Build history of the part. All positions in model axes, mm. A direction names the side the tool comes from. Coordinates: 2 decimals unless noted, no trailing zeros. Order: outer loops, then holes, each group sorted by start corner. A loop starts at its lowest first (then second) coordinate and runs counter-clockwise, first axis right, second up. Notation, with made-up numbers: (71.5, 70.25) -> (110.5, 70.25) arc R23 cw to (110.5, 105.25) -> close; hole circle Ø11 at (-5.5, 25). An arc over 180 degrees is marked (long way). Write each question's results on one line, items separated by ' | '.
from build123d import *

# Parameters (mm, degrees)
EXTRUDE_1_DEPTH = 21.5
SKETCH_2_W      = 9.5
SKETCH_2_H      = 12
EXTRUDE_2_DEPTH = 5
SKETCH_3_W      = 10
SKETCH_3_H      = 12
EXTRUDE_3_DEPTH = 9
SKETCH_4_R      = 2
EXTRUDE_4_DEPTH = 0.7
EXTRUDE_6_DEPTH = 9.3


with BuildPart() as part:
    # 草图1 → 凸台-拉伸1 (new body)
    with BuildSketch(Plane(origin=(0, 0, 0), x_dir=(1, 0, 0), z_dir=(0, 1, 0))):
        with BuildLine():
            Line((-5, -3.31662479), (-5, 3.31662479))
            ThreePointArc((-5, 3.31662479), (0, 6), (5, 3.31662479))
            Line((5, 3.31662479), (5, -3.31662479))
            ThreePointArc((5, -3.31662479), (0, -6), (-5, -3.31662479))
        make_face()
    extrude(amount=EXTRUDE_1_DEPTH)

    # 草图2 → 凸台-拉伸2 (add)
    with BuildSketch(Plane(origin=(0, 21.5, 0), x_dir=(1, 0, 0), z_dir=(0, 1, 0))):
        with Locations((4.75, 0)):
            Rectangle(SKETCH_2_W, SKETCH_2_H)
    extrude(amount=-EXTRUDE_2_DEPTH)

    # 草图3 → 凸台-拉伸3 (add)
    with BuildSketch(Plane.XZ):
        Rectangle(SKETCH_3_W, SKETCH_3_H)
    extrude(amount=EXTRUDE_3_DEPTH)

    # 草图4 → 凸台-拉伸4 (add)
    with BuildSketch(Plane.XZ.offset(9)):
        with Locations(Location((0, 0, 0), (0, 0, 270))):
            Circle(SKETCH_4_R)
    extrude(amount=EXTRUDE_4_DEPTH)

    # 草图5 → 凸台-拉伸6 (add)
    with BuildSketch(Plane.XZ.offset(9.7)):
        with BuildLine():
            Line((-1.118033989, 1), (1.118033989, 1))
            ThreePointArc((1.118033989, 1), (0, -1.5), (-1.118033989, 1))
        make_face()
    extrude(amount=EXTRUDE_6_DEPTH)


solid = part.part
Item 1: Pull direction Y, two halves, no side cores. Call faces 6 (the flat face through (5, 19, -6)), 7 (the flat face through (4, 0, 5)), 8 (the flat face through (-4, 0, 5)): released by +Y, released by -Y, zero draft, split by the parting line, or undercut.
Answer:
face 6: zero draft | face 7: undercut | face 8: released by +Y
Item 2: Drill centre lines: line 1 (Y direction, x = 4.5, z = 4.75); line 2 (X direction, y = 18.5, z = -5); line 3 (Y direction, x = -1.75, z = 0.5). Where is each one in solid material? Low to high. Write a range as from..to.
Answer:
line 1: y = -9..0, 16.5..21.5 | line 2: x = -3.32..9.5 | line 3: y = -9.7..21.5
Item 3: Slice it at B-B, the plane y = -6. List the corners of the cut face in (x, z).
Answer:
outline: (-5, -6) -> (5, -6) -> (5, 6) -> (-5, 6) -> close
Item 4: Slice it at C-C, the plane x = 6. List the corners of the cut face in (y, z).
Answer:
outline: (16.5, -6) -> (21.5, -6) -> (21.5, 6) -> (16.5, 6) -> close
Item 5: Slice it at D-D, the plane z = 2.5. List the corners of the cut face in (x, y).
Answer:
outline: (-5, -9) -> (5, -9) -> (5, 16.5) -> (9.5, 16.5) -> (9.5, 21.5) -> (-5, 21.5) -> close
Item 6: Tool access for faces 1 (the flat face through (-4, 0, -5)), 2 (the cylindrical face through (0, 11, -6)), 3 (the cylindrical face through (0, 11, 6)), 4 (the flat face through (0, -14, 1)), 5 (the cylindrical face through (-1.952, -9.345, 0.434)): list every direction of +Z, -Z, +X, -X, +Y, -Y with a clear straight run to the whole face (end or side of a thin tool).
Answer:
face 1: -Z, -X, +Y | face 2: -Z | face 3: +Z | face 4: +Z, +X, -X, -Y | face 5: -Y
Item 7: Slice it at A-A, the plane z = 0. List the corners of the cut face in (x, y), and give its area (3 significant figures).
Answer:
outline: (-5, -9) -> (-2, -9) -> (-2, -9.7) -> (-1.5, -9.7) -> (-1.5, -19) -> (1.5, -19) -> (1.5, -9.7) -> (2, -9.7) -> (2, -9) -> (5, -9) -> (5, 16.5) -> (9.5, 16.5) -> (9.5, 21.5) -> (-5, 21.5) -> close | area: 358 mm^2
Item 8: Pin check, flat tips, straight feed: pin 1 (0.7 mm diameter, centred on x = -0.5, y = -15.5, fed in from +Z); pin 2 (1 mm diameter, centred on y = -2.5, z = -3.5, fed in from +X); pin 3 (3 mm diameter, centred on x = -0.5, y = 9.5, fed in from +Z); pin 4 (2 mm diameter, centred on x = 5.5, y = 7.5, fed in from +Z). Stop position of each tip, or through.
Answer:
pin 1: stops at z = 1 | pin 2: stops at x = 5 | pin 3: stops at z = 6 | pin 4: stops at z = 3.97
